Design review of the part built by this model. Coordinates are the model's own, in mm. Coordinates: 2 decimals unless noted, no trailing zeros. Loops run counter-clockwise (first coordinate to the right, second up) from the corner with the lowest first, then second, coordinate; pieces in that order, holes last.
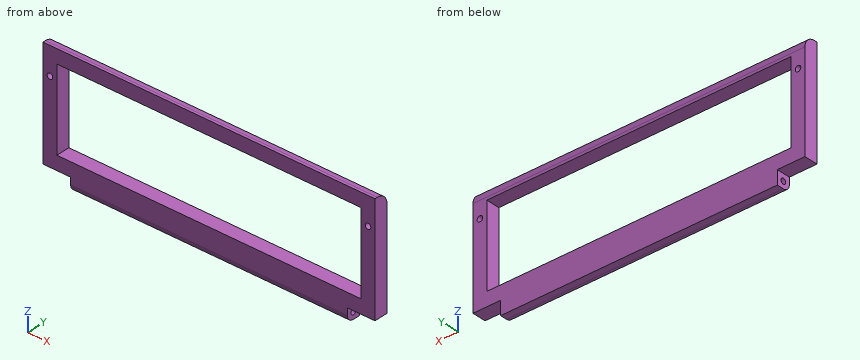
from build123d import *

# Parameters (mm, degrees)
F1_DEPTH = 6.35
F2_R     = 3.175
F3_R     = 1.27
F4_DEPTH = 139.701
F5_R     = 5.08
F6_R     = 1.27
F7_DEPTH = 6.351


with BuildPart() as f1:
    # F0 (on Front) → F1 (new body)
    with BuildSketch(Plane.XZ):
        Polygon((152.4, 0), (0, 0), (0, -50.292001), (12.7, -50.292001), (12.7, -56.642), (139.7, -56.642), (139.7, -50.292001), (152.4, -50.292001), align=None)
        Polygon((146.05, -6.35), (146.05, -43.942001), (139.7, -43.942001), (12.7, -43.942001), (6.35, -43.942001), (6.35, -6.35), align=None, mode=Mode.SUBTRACT)
    extrude(amount=-F1_DEPTH)

    # F2
    f2_edges = [f1.edges().sort_by_distance(p)[0] for p in [
        (76.2, 0, -56.642),
    ]]
    fillet(f2_edges, radius=F2_R)

    # F3 (on face) → F4 (cut, through all)
    with BuildSketch(Plane(origin=(12.7, 0, 0), x_dir=(0, -1, 0), z_dir=(-1, 0, 0))):
        with Locations((-3.175, -53.467)):
            Circle(F3_R)
    extrude(amount=-F4_DEPTH, mode=Mode.SUBTRACT)

    # F5
    f5_edges = [f1.edges().sort_by_distance(p)[0] for p in [
        (76.2, 6.35, 0),
    ]]
    fillet(f5_edges, radius=F5_R)

    # F6 (on face) → F7 (cut, through all)
    with BuildSketch(Plane(origin=(0, 6.35, 0), x_dir=(-1, 0, 0), z_dir=(0, 1, 0))):
        with Locations((-149.225, -12.7)):
            Circle(F6_R)
        with Locations((-3.175, -12.7)):
            Circle(F6_R)
    extrude(amount=-F7_DEPTH, mode=Mode.SUBTRACT)


solid = f1.part
Q1. Clearance check with flat-ended pins moving along their axes: pin 1 Ø1.5 at (x, y) = (134.5, 0.5) entering from -Z; pin 2 Ø3 at (x, y) = (145.5, 3) entering from -Z; pin 3 Ø3 at (y, z) = (4, -53) entering from +X. State where each tip first meets the part, or that it passes through.
Q2. Take a section at A-A, the plane x = 77. Write out the cut boundary in (y, z) (3 decimals).
Q3. For line 1 (X direction, y = 4.25, z = -12); line 2 (Z direction, x = 114, y = 2.5); line 3 (X direction, y = 2.25, z = -8.5), list the stretches that pass through material, from the lowest coordinate up.
Q4. Take a section at B-B, the plane z = -8. Write out the cut boundary in (x, y), then the cut area to 3 significant figures.
Entries:
1. pin 1: stops at z = -55.99
1. pin 2: stops at z = -50.29
1. pin 3: stops at x = 139.7
2. outline: (0, -53.467) arc R3.175 ccw to (3.175, -56.642) - (6.35, -56.642) - (6.35, -43.942) - (0, -43.942) - close; (0, -6.35) - (6.35, -6.35) - (6.35, -5.08) arc R5.08 ccw to (1.27, 0) - (0, 0) - close; hole circle Ø2.54 at (3.175, -53.467)
3. line 1: x = 0 to 2.12, 4.23 to 6.35, 146.05 to 148.17, 150.28 to 152.4
3. line 2: z = -56.57 to -54.54, -52.39 to -43.94, -6.35 to -0.15
3. line 3: x = 0 to 6.35, 146.05 to 152.4
4. outline: (0, 0) - (6.35, 0) - (6.35, 6.35) - (0, 6.35) - close; (146.05, 0) - (152.4, 0) - (152.4, 6.35) - (146.05, 6.35) - close
4. area: 80.6 mm2
